Here's how the part is built. I have some questions about the finished solid (model axes, mm). Coordinates: 2 decimals unless noted, no trailing zeros. Answer as a JSON object with one key per item and string values. Group by question number.
1) I'm going to push a flat-ended pin straight in: pin 1 (2 mm diameter, centred on x = 134.5, z = 1.5, fed in from -Y). Where does the tip first touch, or does it pass through?
2) I want a section at C-C (z = 8). Count the separate pieces of the cut face and the enclosed holes in it, then the cut area to 3 significant figures.
3) I need wall thicknesses on probe 1 along Y at (x, z) = (207.5, 9.25); probe 2 along Y at (x, z) = (123, 9.75); probe 3 along Y at (x, z) = (74.5, 6.5). Which ranges of each line are inside material? Lowest first, please. Write a range as [from, to].
```python
from build123d import *

# Parameters (mm, degrees)
ESQUISSE1_W             = 424
ESQUISSE1_H             = 850
BOSS_EXTRU_1_DEPTH      = 10
ENL_V_MAT_EXTRU_1_DEPTH = 5
CHANFREIN1_SIZE         = 5


with BuildPart() as part:
    # Esquisse1 → Boss.-Extru.1 (new body)
    with BuildSketch(Plane.XY):
        with Locations((212, 425)):
            Rectangle(ESQUISSE1_W, ESQUISSE1_H)
    extrude(amount=BOSS_EXTRU_1_DEPTH)

    # Esquisse2 → Enlèv. mat.-Extru.1 (cut)
    with BuildSketch(Plane.XY.offset(10)):
        Polygon((100, 231.923881554), (100, 618.076118446), (40, 678.076118446), (40, 171.923881554), align=None)
        Polygon((191.923881554, 710), (232.076118446, 710), (332.076118446, 810), (91.923881554, 810), align=None)
        Polygon((40, 810), (40, 720.502525317), (130, 630.502525317), (130, 219.497474683), (40, 129.497474683), (40, 40), (49.497474683, 40), (179.497474683, 170), (244.502525317, 170), (374.502525317, 40), (384, 40), (384, 129.497474683), (294, 219.497474683), (294, 630.502525317), (384, 720.502525317), (384, 810), (374.502525317, 810), (244.502525317, 680), (179.497474683, 680), (49.497474683, 810), align=None)
        Polygon((324, 231.923881554), (324, 618.076118446), (384, 678.076118446), (384, 171.923881554), align=None)
        Polygon((332.076118446, 40), (91.923881554, 40), (191.923881554, 140), (232.076118446, 140), align=None)
    extrude(amount=-ENL_V_MAT_EXTRU_1_DEPTH, mode=Mode.SUBTRACT)

    # Chanfrein1
    chanfrein1_edges = [part.edges().sort_by_distance(p)[0] for p in [
        (212, 40, 5),
        (141.923881554, 90, 5),
        (212, 140, 5),
        (282.076118446, 90, 5),
        (40, 425, 5),
        (70, 648.076118446, 5),
        (100, 425, 5),
        (70, 201.923881554, 5),
        (384, 425, 5),
        (354, 201.923881554, 5),
        (324, 425, 5),
        (354, 648.076118446, 5),
        (114.497474683, 745, 5),
        (212, 680, 5),
        (309.502525317, 745, 5),
        (379.251262658, 810, 5),
        (384, 765.251262658, 5),
        (339, 675.502525317, 5),
        (294, 425, 5),
        (339, 174.497474683, 5),
        (384, 84.748737342, 5),
        (379.251262658, 40, 5),
        (309.502525317, 105, 5),
        (212, 170, 5),
        (114.497474683, 105, 5),
        (44.748737342, 40, 5),
        (40, 84.748737342, 5),
        (85, 174.497474683, 5),
        (130, 425, 5),
        (85, 675.502525317, 5),
        (40, 765.251262658, 5),
        (44.748737342, 810, 5),
        (212, 810, 5),
        (282.076118446, 760, 5),
        (212, 710, 5),
        (141.923881554, 760, 5),
    ]]
    chamfer(chanfrein1_edges, length=CHANFREIN1_SIZE - 0.0001)  # a hair under: the kernel refuses the full size


solid = part.part
```
Determined:
{
 "1": {"pin 1": "y = 0"},
 "2": {"separate pieces": "1", "enclosed holes": "5", "area": "166,000 mm^2"},
 "3": {"probe 1": "[0, 40.75], [139.25, 170.75], [679.25, 710.75], [809.25, 850]", "probe 2": "[0, 40.25], [70.72, 113.86], [212.14, 637.86], [736.14, 779.28], [809.75, 850]", "probe 3": "[0, 69.95], [159.05, 211.37], [638.63, 690.95], [780.05, 850]"}
}
